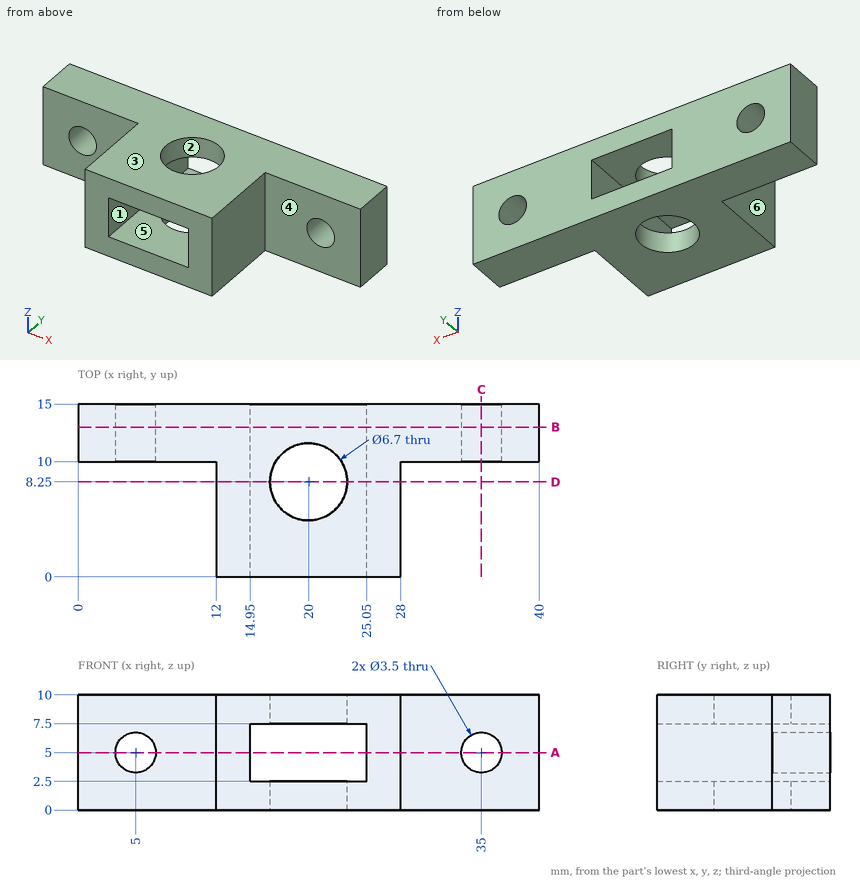
Study the drawing (mm; zero at the part's minimum x, y, z) and answer. A direction names the side the tool comes from. Give positions to 0.01 mm unless a question says otherwise; leave off trailing zeros. Write each loop counter-clockwise with the first axis right and the second up, starting at its lowest first coordinate (ties: lowest second). Pieces come first, ordered by that corner, then holes. Notation, with made-up numbers: (-36.75, 12) -> (-26.75, 12) arc R14 ccw to (-26.75, 34) -> close; hole circle Ø6 at (59, -31). An arc over 180 degrees is marked (long way). Write item = value, one per line.
Q1. Flat-ended cylindrical pins translate along their axes: pin 1 Ø4 at (y, z) = (7, 5) entering from -X; pin 2 Ø1.5 at (x, z) = (6, 1.5) entering from -Y. Find the tip coordinate at first contact, or state that the pin passes through.
Computed values:
pin_1 = 12
pin_2 = 10
Q2. Section B-B on y = 13 is taken. Determine the outline of the cut face in (x, z), and give its area (3 significant figures).
Computed values:
outline = (0, 0) -> (40, 0) -> (40, 10) -> (0, 10) -> close; hole circle Ø3.5 at (5, 5); hole (14.95, 2.5) -> (25.05, 2.5) -> (25.05, 7.5) -> (14.95, 7.5) -> close; hole circle Ø3.5 at (35, 5)
area = 330 mm^2
Q3. A tool of negligible diameter and unlimited length cuts with its end or side. For the marked faces 4, 5 and 6, from which of +Z, -Z, +X, -X, +Y, -Y can it reach the whole face along a straight path? Write none if from no direction.
Computed values:
face_4 = +Z, -Z, +X, -Y
face_5 = +Y, -Y
face_6 = +Z, -Z, -X, -Y
Q4. For a pull along Z with two mould halves and no side action, classify the marked faces 1, 2 and 3 as pulls with the +Z half, pulls with the -Z half, needs draft (parallel to the pull), parting line crosses it, or undercut.
Computed values:
face_1 = undercut
face_2 = needs draft
face_3 = pulls with the +Z half
Q5. Consider line 1 along Z through (x, y) = (16, 5.75); line 2 along X through (y, z) = (8.25, 9.2); line 3 along Y through (x, z) = (20, 9.1). Determine where each line is inside the solid, lowest interval first.
Computed values:
line_1 = 0 to 2.5, 7.5 to 10
line_2 = 12 to 16.65, 23.35 to 28
line_3 = 0 to 4.9, 11.6 to 15
Q6. Section C-C on x = 35 is taken. Determine the outline of the cut face in (y, z).
Computed values:
outline = (10, 0) -> (15, 0) -> (15, 3.25) -> (10, 3.25) -> close; (10, 6.75) -> (15, 6.75) -> (15, 10) -> (10, 10) -> close
Q7. Section D-D on y = 8.25 is taken. Determine the outline of the cut face in (x, z).
Computed values:
outline = (12, 0) -> (16.65, 0) -> (16.65, 2.5) -> (14.95, 2.5) -> (14.95, 7.5) -> (16.65, 7.5) -> (16.65, 10) -> (12, 10) -> close; (23.35, 0) -> (28, 0) -> (28, 10) -> (23.35, 10) -> (23.35, 7.5) -> (25.05, 7.5) -> (25.05, 2.5) -> (23.35, 2.5) -> close
Q8. Section A-A on z = 5 is taken. Determine the outline of the cut face in (x, y).
Computed values:
outline = (0, 10) -> (3.25, 10) -> (3.25, 15) -> (0, 15) -> close; (6.75, 10) -> (12, 10) -> (12, 0) -> (14.95, 0) -> (14.95, 15) -> (6.75, 15) -> close; (25.05, 0) -> (28, 0) -> (28, 10) -> (33.25, 10) -> (33.25, 15) -> (25.05, 15) -> close; (36.75, 10) -> (40, 10) -> (40, 15) -> (36.75, 15) -> close
